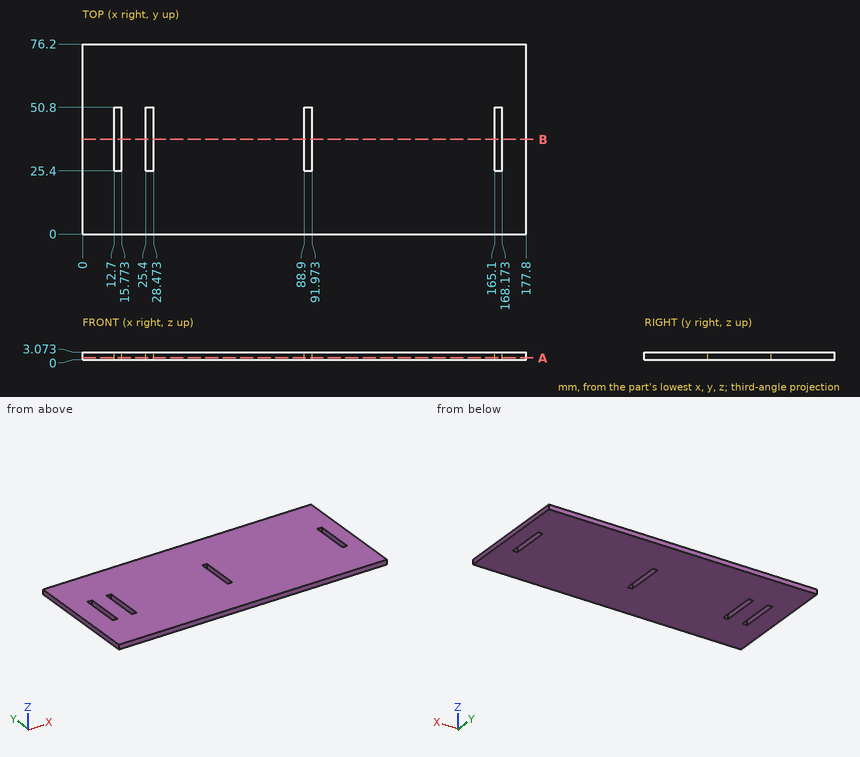
Check sheet for the drawn part. Datum: minimum x, y, z corner. Units: mm. Round coordinates to 2 decimals unless told otherwise and drop trailing zeros. Order: outer loops, then holes, each group sorted by start corner. A loop starts at its lowest first (then second) coordinate and runs counter-clockwise, first axis right, second up. Notation, with made-up numbers: (68, 32.5) - (90, 32.5) arc R28 cw to (90, 61.5) - close; hole circle Ø10 at (64, 64.5). An arc over 180 degrees is marked (long way). Use a Markdown table: item, result. Add a question column.
(1) Material ranges on line 1 along X through (y, z) = (35, 0.6); line 2 along Y through (x, z) = (26, 1.25), recorded low to high. Write a range as [from, to].
(2) Sectioned sample at B-B, the plane y = 38. Enter the section's corners in (x, z).
(3) Sectioned sample at A-A, the plane z = 0.75. Enter the section's corners in (x, y), and give its area (3 significant figures).
Answers below:
| question | item | result |
|---|---|---|
| 1 | line 1 | [0, 12.7], [15.77, 25.4], [28.47, 88.9], [91.97, 165.1], [168.17, 177.8] |
| 1 | line 2 | [0, 25.4], [50.8, 76.2] |
| 2 | outline | (0, 0) - (12.7, 0) - (12.7, 3.07) - (0, 3.07) - close; (15.77, 0) - (25.4, 0) - (25.4, 3.07) - (15.77, 3.07) - close; (28.47, 0) - (88.9, 0) - (88.9, 3.07) - (28.47, 3.07) - close; (91.97, 0) - (165.1, 0) - (165.1, 3.07) - (91.97, 3.07) - close; (168.17, 0) - (177.8, 0) - (177.8, 3.07) - (168.17, 3.07) - close |
| 3 | outline | (0, 0) - (177.8, 0) - (177.8, 76.2) - (0, 76.2) - close; hole (12.7, 25.4) - (15.77, 25.4) - (15.77, 50.8) - (12.7, 50.8) - close; hole (25.4, 25.4) - (28.47, 25.4) - (28.47, 50.8) - (25.4, 50.8) - close; hole (88.9, 25.4) - (91.97, 25.4) - (91.97, 50.8) - (88.9, 50.8) - close; hole (165.1, 25.4) - (168.17, 25.4) - (168.17, 50.8) - (165.1, 50.8) - close |
| 3 | area | 13,200 mm² |
